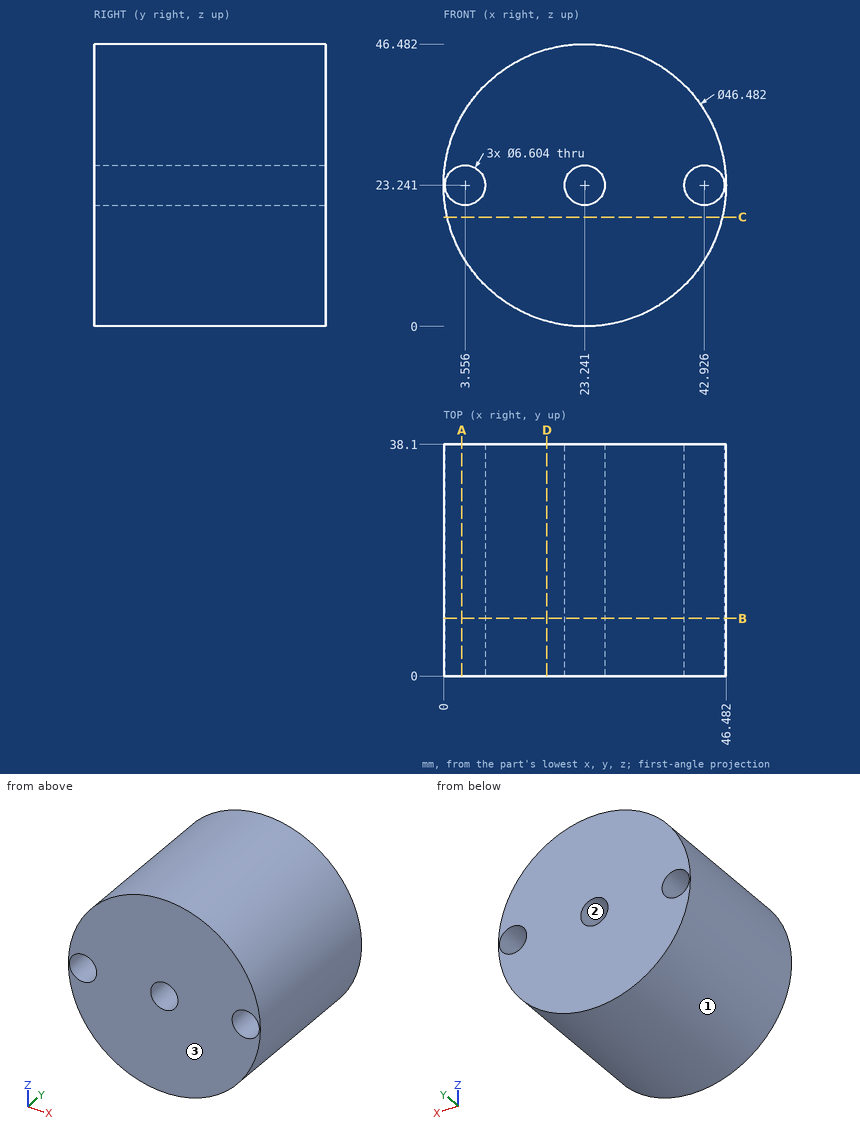
Can you work these out from the drawing? Everything is in mm from the part's minimum corner. Give positions to 0.01 mm unless a question says otherwise; leave off trailing zeros. Loops run counter-clockwise (first coordinate to the right, second up) from the corner with the lowest first, then second, coordinate; pieces in that order, holes last. Notation, with made-up numbers: M 78,40 L 98,40 A19 ccw 98,74 Z; hole C 28.5,4 d3. An arc over 180 degrees is marked long. Put each result on its own line as item: value. Start each with the question number.
(1) I want a section at A-A on x = 3. Please give me the cut outline in (y, z), then the cut area to 3 significant figures.
(2) Will these pins go through, and if not, where does the flat tip stop? pin 1 Ø4 at (x, z) = (27, 29) entering from -Y; pin 2 Ø1 at (x, y) = (25, 16) entering from -Z; pin 3 Ø5.5 at (x, z) = (3.556, 23.241) entering from +Y; pin 4 Ø3 at (x, y) = (35.5, 33) entering from +Z.
(3) I want a section at B-B on y = 9.5. Please give me the cut outline in (x, z), then the cut area to 3 significant figures.
(4) I need wall thicknesses on line 1 along X through (y, z) = (22, 20.5); line 2 along Z through (x, y) = (21.5, 34); line 3 along Z through (x, y) = (22.5, 34). Which ranges of each line are inside material? Lowest first, please. Write a range as [from, to].
(5) I want a section at C-C on z = 18. Please give me the cut outline in (x, y), then the cut area to 3 significant figures.
(6) If we mould it in two halves opening along X, with no side actions, what happens to the marked faces 1, 2 and 3? For each: +X half, -X half, draft (parallel to the pull), parting line (faces both ways), or undercut.
(7) I want a section at D-D on x = 17. Please give me the cut outline in (y, z), then the cut area to 3 significant figures.
Answer block:
1. outline: M 0,11.82 L 38.1,11.82 L 38.1,19.99 L 0,19.99 Z; M 0,26.5 L 38.1,26.5 L 38.1,34.66 L 0,34.66 Z
1. area: 622 mm^2
2. pin 1: y = 0
2. pin 2: z = 0.03
2. pin 3: through
2. pin 4: z = 43.84
3. outline: C 23.24,23.24 d46.48; hole C 3.56,23.24 d6.6; hole C 23.24,23.24 d6.6; hole C 42.93,23.24 d6.6
3. area: 1,590 mm^2
4. line 1: [0.16, 1.71], [5.4, 21.4], [25.08, 41.08], [44.77, 46.32]
4. line 2: [0.07, 20.44], [26.05, 46.42]
4. line 3: [0.01, 20.02], [26.46, 46.47]
5. outline: M 0.6,0 L 45.88,0 L 45.88,38.1 L 0.6,38.1 Z
5. area: 1,730 mm^2
6. face 1: parting line
6. face 2: undercut
6. face 3: draft
7. outline: M 0,0.85 L 38.1,0.85 L 38.1,45.63 L 0,45.63 Z
7. area: 1,710 mm^2
